Geometry: final body of the model. Coordinates: model frame, mm. A direction names the side the tool comes from. Give positions to 0.01 mm unless a question says otherwise; leave off trailing zeros. Order: outer loops, then holes, each group sorted by start corner. A loop starts at its lowest first (then second) coordinate and runs counter-clockwise, first axis right, second up. Notation, with made-up numbers: (78, 82) -> (89, 82) arc R20 cw to (89, 120) -> close; hole circle Ø7 at (51.5, 89.5). An arc over 180 degrees is marked (long way). One line per question, with ' | ' between items. Start each with the question number.
(1) Mould query, pull axis Y, two halves, no side actions, for faces 1 (the face through (5.334, 97, 2)), 2 (the face through (0, 106.375, 0)), 3 (the face through (-5.334, 99, 0)). Classes: +Y half, -Y half, draft (parallel to the pull), parting line (faces both ways), or undercut.
(2) First-contact query: pin 1 Ø2 at (x, y) = (-2, 55.5) entering from -Z; pin 2 Ø4.5 at (y, z) = (97, -1.5) entering from +X; pin 3 Ø1.9 at (x, z) = (1, 0.5) entering from -Y; pin 4 Ø4.5 at (y, z) = (98, -5.5) entering from +X. Flat tips, straight axial feed; report the tip coordinate or a pass-through.
(3) Set-up query: faces 4 (the face through (0, 99, 18.977)), 5 (the face through (-0.41, 45.37, -3.15)), 6 (the face through (-0.797, 63.115, 3.588)), 7 (the face through (5.334, 97.1, -4.5)). Return all of +Z, -Z, +X, -X, +Y, -Y with unobstructed straight access to the full face (end or side cutting, diameter ignored); none if empty.
(4) Section A-A (y = 56). Return loops of the section in (x, z) (3 decimals), then the cut area to 3 significant figures.
(5) Section C-C (z = -12). Return loops of the section in (x, y).
(6) Ray query, L1, parallel to X at y = 60.5, z = 0 (3 decimals); L2, parallel to Z at x = -0.5, y = 40. Return the intervals inside material, ascending.
(7) Section B-B (x = -1.5). Return loops of the section in (y, z), then the cut area to 3 significant figures.
```python
from build123d import *

# Parameters (mm, degrees)
SKETCH2_R            = 36.75
SKETCH2_R_2          = 31.75
BOSS_EXTRUDE2_DEPTH  = 900
BOSS_EXTRUDE10_DEPTH = 5
CIRPATTERN3_COUNT    = 4
SKETCH5_R            = 44.75
SKETCH5_R_2          = 36.75
BOSS_EXTRUDE11_DEPTH = 10
LPATTERN1_COUNT      = 2
LPATTERN1_PITCH      = 80
BOSS_EXTRUDE12_DEPTH = 53.34
SKETCH7_R            = 46.138276775
SKETCH7_R_2          = 35.802049151
BOSS_EXTRUDE15_DEPTH = 55.372
SKETCH8_R            = 20.14340108
BOSS_EXTRUDE16_DEPTH = 55.372
SKETCH9_R            = 5.663284778
BOSS_EXTRUDE18_DEPTH = 55.88
SCALE1_SCALE         = 0.1


with BuildPart() as part:
    # Sketch2 → Boss-Extrude2 (new body)
    with BuildSketch(Plane(origin=(0, 10, 0), x_dir=(1, 0, 0), z_dir=(0, 1, 0))):
        Circle(SKETCH2_R)
        Circle(SKETCH2_R_2, mode=Mode.SUBTRACT)
    extrude(amount=BOSS_EXTRUDE2_DEPTH)

    # Sketch5 → Boss-Extrude11 (add)
    with BuildSketch(Plane(origin=(0, 280.000000004, 0), x_dir=(1, 0, 0), z_dir=(0, 1, 0))):
        Circle(SKETCH5_R)
        Circle(SKETCH5_R_2, mode=Mode.SUBTRACT)
    boss_extrude11 = extrude(amount=-BOSS_EXTRUDE11_DEPTH)

    # LPattern1: Boss-Extrude11 ×2
    with Locations(*[(0, i * LPATTERN1_PITCH, 0) for i in range(1, LPATTERN1_COUNT)]):
        add(boss_extrude11)

    # Sketch6 → Boss-Extrude12 (add, symmetric)
    with BuildSketch(Plane(origin=(0, 0, 0), x_dir=(0, 0, -1), z_dir=(1, 0, 0))):
        Polygon((-36.75, 910), (-189.768574018, 910), (-189.768574018, 1063.746484801), (189.768574018, 1063.746484801), (189.768574018, 910), (36.75, 910), align=None)
    extrude(amount=BOSS_EXTRUDE12_DEPTH, both=True)

    # Sketch7 → Boss-Extrude15 (add)
    with BuildSketch(Plane(origin=(0, 0, 0), x_dir=(0, 0, -1), z_dir=(1, 0, 0))):
        with Locations((0, 986.650763521)):
            Circle(SKETCH7_R)
        with Locations((0, 986.650763521)):
            Circle(SKETCH7_R_2, mode=Mode.SUBTRACT)
    extrude(amount=BOSS_EXTRUDE15_DEPTH)

    # Sketch8 → Boss-Extrude16 (add)
    with BuildSketch(Plane(origin=(0, 0, 0), x_dir=(0, 0, -1), z_dir=(1, 0, 0))):
        with Locations((0, 986.650763521)):
            Circle(SKETCH8_R)
    extrude(amount=BOSS_EXTRUDE16_DEPTH)

    # Sketch9 → Boss-Extrude18 (add)
    with BuildSketch(Plane(origin=(0, 0, 0), x_dir=(0, 0, -1), z_dir=(1, 0, 0))):
        with Locations((0, 986.650763521)):
            Circle(SKETCH9_R)
    extrude(amount=BOSS_EXTRUDE18_DEPTH)


with BuildPart() as body_2:
    # Sketch4 → Boss-Extrude10 (new body, symmetric)
    with BuildSketch(Plane.XY):
        Polygon((-125, 10), (-125, 37.123747586), (-87.807861708, 71.973477342), (-36.75, 71.973477342), (-36.75, 10), align=None)
    extrude(amount=BOSS_EXTRUDE10_DEPTH, both=True)


with BuildPart() as cirpattern3_1:
    # CirPattern3: pattern copy
    add(body_2.part.rotate(Axis((0, 0, 0), (0, 1, 0)), 1 * 360 / CIRPATTERN3_COUNT))


with BuildPart() as cirpattern3_2:
    # CirPattern3: pattern copy
    add(body_2.part.rotate(Axis((0, 0, 0), (0, 1, 0)), 2 * 360 / CIRPATTERN3_COUNT))


with BuildPart() as cirpattern3_3:
    # CirPattern3: pattern copy
    add(body_2.part.rotate(Axis((0, 0, 0), (0, 1, 0)), 3 * 360 / CIRPATTERN3_COUNT))


with BuildPart() as part_1:
    # Scale1: scaled about (0, 0, 0)
    add(part.part.scale(SCALE1_SCALE))


solid = part_1.part
```
Response:
1) face 1: undercut | face 2: +Y half | face 3: draft
2) pin 1: stops at z = -3.54 | pin 2: stops at x = 5.59 | pin 3: stops at y = 91 | pin 4: stops at x = 5.54
3) face 4: +Z, +X, -X, +Y, -Y | face 5: -Y | face 6: none | face 7: +X
4) outline: circle Ø7.35 at (0, 0); hole circle Ø6.35 at (0, 0) | area: 10.8 mm^2
5) outline: (-5.33, 91) -> (5.33, 91) -> (5.33, 106.37) -> (-5.33, 106.37) -> close
6) L1: x = -3.675 to -3.175, 3.175 to 3.675 | L2: z = -3.64 to -3.14, 3.14 to 3.64
7) outline: (1, -3.35) -> (27, -3.35) -> (27, -4.22) -> (28, -4.22) -> (28, -3.35) -> (35, -3.35) -> (35, -4.22) -> (36, -4.22) -> (36, -3.35) -> (91, -3.35) -> (91, -18.98) -> (106.37, -18.98) -> (106.37, 18.98) -> (91, 18.98) -> (91, 3.35) -> (36, 3.35) -> (36, 4.22) -> (35, 4.22) -> (35, 3.35) -> (28, 3.35) -> (28, 4.22) -> (27, 4.22) -> (27, 3.35) -> (1, 3.35) -> (1, 2.8) -> (91, 2.8) -> (91, -2.8) -> (1, -2.8) -> close | area: 687 mm^2
